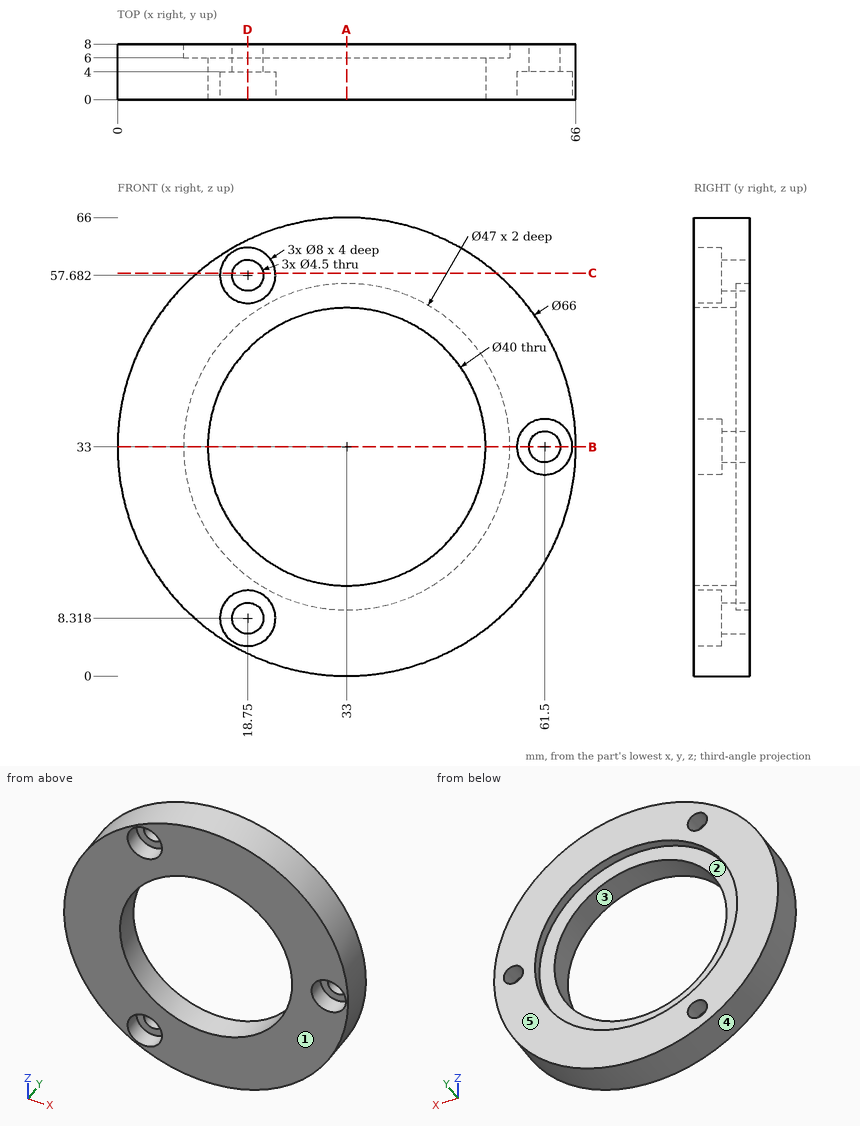
Answer from the drawing. Dimensions are ordinates in mm from the lowest x, y and z of the part. A direction names the side the tool comes from. Coordinates: 2 decimals unless noted, no trailing zeros. Write each loop counter-clockwise with the first axis right and the second up, starting at its lowest first coordinate (ties: lowest second). Pieces come first, ordered by that corner, then holes. Notation, with made-up numbers: M 86,34.5 L 133,34.5 A15 ccw 133,51.5 Z; hole C 52,1.5 d10. An arc over 180 degrees is marked long. Write item = value, one per line.
1. The part is cut by section A-A (x = 33). Determine the outline of the cut face in (y, z), then the cut area to 3 significant figures.
Solution:
outline = M 0,0 L 8,0 L 8,9.5 L 6,9.5 L 6,13 L 0,13 Z; M 0,53 L 6,53 L 6,56.5 L 8,56.5 L 8,66 L 0,66 Z
area = 194 mm2
2. The part is cut by section B-B (z = 33). Determine the outline of the cut face in (x, y).
Solution:
outline = M 0,0 L 13,0 L 13,6 L 9.5,6 L 9.5,8 L 0,8 Z; M 53,0 L 57.5,0 L 57.5,4 L 59.25,4 L 59.25,8 L 56.5,8 L 56.5,6 L 53,6 Z; M 63.75,4 L 65.5,4 L 65.5,0 L 66,0 L 66,8 L 63.75,8 Z
3. For the marked faces 1 and 2, determine the directions among +Z, -Z, +X, -X, +Y, -Y from which every point of the face is accessible in a straight line to the end or side of a thin tool.
Solution:
face_1 = +Z, -Z, +X, -X, -Y
face_2 = +Y
4. Determine the mould class of the marked faces 3, 4 and 5 for opening direction Z: released by +Z, released by -Z, zero draft, split by the parting line, or undercut.
Solution:
face_3 = undercut
face_4 = split by the parting line
face_5 = zero draft
5. Flat-ended cylindrical pins translate along their axes: pin 1 (2.5 mm diameter, centred on x = 20.5, z = 59, fed in from -Y); pin 2 (3 mm diameter, centred on x = 22, y = 6, fed in from -Z); pin 3 (2 mm diameter, centred on x = 18, y = 4, fed in from -Z). Find the tip coordinate at first contact, or state that the pin passes through.
Solution:
pin_1 = 4
pin_2 = 1.4
pin_3 = 3.12
6. Straight lines are drawn through the part: line 1 (Z direction, x = 18.75, y = 5.8) (1 decimal); line 2 (Z direction, x = 33.5, y = 1.25); line 3 (Z direction, x = 61.5, y = 1.3) (1 decimal). For each, find the intervals that lie inside material, in ascending order. Write a range as from..to.
Solution:
line_1 = 3.2..6.1, 10.6..19, 47..55.4, 59.9..62.8
line_2 = 0..13.01, 52.99..66
line_3 = 16.4..29, 37..49.6
7. The part is cut by section C-C (z = 58). Determine the outline of the cut face in (x, y).
Solution:
outline = M 11.46,0 L 14.76,0 L 14.76,4 L 16.52,4 L 16.52,8 L 11.46,8 Z; M 20.98,4 L 22.74,4 L 22.74,0 L 54.54,0 L 54.54,8 L 20.98,8 Z
8. The part is cut by section D-D (x = 18.75). Determine the outline of the cut face in (y, z) (1 decimal).
Solution:
outline = M 0,3.2 L 8,3.2 L 8,6.1 L 4,6.1 L 4,4.3 L 0,4.3 Z; M 0,12.3 L 4,12.3 L 4,10.6 L 8,10.6 L 8,14.3 L 6,14.3 L 6,19 L 0,19 Z; M 0,47 L 6,47 L 6,51.7 L 8,51.7 L 8,55.4 L 4,55.4 L 4,53.7 L 0,53.7 Z; M 0,61.7 L 4,61.7 L 4,59.9 L 8,59.9 L 8,62.8 L 0,62.8 Z
